```python
from build123d import *

# Parameters (mm, degrees)
F1_DEPTH    = 25
F2_R        = 5
F3_T1_DEPTH = 50.8882578448
F3_T3_DEPTH = 49.1422193702
F4_T1_DEPTH = 50.8882578448
F5_R        = 5


# Not quite as in the source:
# - a fillet or chamfer that OpenCascade refuses, or shapes differently, is made with other operations: its cross-section is extruded or revolved along the edge and cut away or added


with BuildPart() as f1:
    # F0 (on Front) → F1 (new body)
    with BuildSketch(Plane.XZ):
        Polygon((-29.6450223361, 14.0248785508), (-30, 3.8596482585), (-20, 3.8596482585), (-19.6450223361, 14.0248785508), align=None)
        Polygon((-20, 3.8596482585), (-30, 3.8596482585), (-30, -6.1403517415), (17.9300867021, -6.1403517415), (17.9300867021, 3.8596482585), (0, 3.8596482585), (-10, 3.8596482585), align=None)
        Polygon((-9.3028735371, 23.8227382193), (-10, 3.8596482585), (0, 3.8596482585), (0.6971264629, 23.8227382193), align=None)
    extrude(amount=F1_DEPTH)

    # F2
    f2_edges = [f1.edges().sort_by_distance(p)[0] for p in [
        (-29.645022, -12.5, 14.024879),
    ]]
    fillet(f2_edges, radius=F2_R)

    # F3: fillet of radius 5 on 2 edges, made by hand

    # F3_s2 → F3_t1 (cut)
    with BuildSketch(Plane.XZ.offset(-12.9441289224)):
        with BuildLine():
            ThreePointArc((-24.8226739051, 14.0248785508), (-21.2259749034, 12.4981704031), (-19.82571977, 8.8503810672))
            Line((-19.82571977, 8.8503810672), (-19.6450223361, 14.0248785508))
            Line((-19.6450223361, 14.0248785508), (-24.8226739051, 14.0248785508))
        make_face()
    extrude(amount=F3_T1_DEPTH, mode=Mode.SUBTRACT)

    # F3_s4 → F3_t3 (cut)
    with BuildSketch(Plane.XZ.offset(-12.0711096851)):
        with BuildLine():
            ThreePointArc((-9.4713837982, 18.9972357029), (-7.9477215154, 22.419437221), (-4.4744296631, 23.8227382193))
            Line((-4.4744296631, 23.8227382193), (-9.3028735371, 23.8227382193))
            Line((-9.3028735371, 23.8227382193), (-9.4713837982, 18.9972357029))
        make_face()
    extrude(amount=F3_T3_DEPTH, mode=Mode.SUBTRACT)

    # F4: fillet of radius 5 on 1 edges, made by hand

    # F4_s2 → F4_t1 (cut)
    with BuildSketch(Plane.XZ.offset(-12.9441289224)):
        with BuildLine():
            ThreePointArc((-4.4805251061, 23.8227382193), (-0.8838261044, 22.2960300716), (0.516429029, 18.6482407358))
            Line((0.516429029, 18.6482407358), (0.6971264629, 23.8227382193))
            Line((0.6971264629, 23.8227382193), (-4.4805251061, 23.8227382193))
        make_face()
    extrude(amount=F4_T1_DEPTH, mode=Mode.SUBTRACT)

    # F5
    f5_edges = [f1.edges().sort_by_distance(p)[0] for p in [
        (17.930087, -12.5, 3.859648),
    ]]
    fillet(f5_edges, radius=F5_R)


solid = f1.part
```
Verification items for the finished model (mm, model axes). Coordinates: 2 decimals unless noted, no trailing zeros. Loops run counter-clockwise (first coordinate to the right, second up) from the corner with the lowest first, then second, coordinate; pieces in that order, holes last. Notation, with made-up numbers: (-8, 70) - (44, 70) arc R19 ccw to (44, 101) - close; hole circle Ø11 at (-33.75, 23.5). An arc over 180 degrees is marked (long way). Put each result on its own line as item: value.
Item 1: Draft check along X on faces 1 (the face through (-6, -12, -6.14)), 2 (the face through (-15, -12, 3.86)), 3 (the face through (-30, -12, -1)), 4 (the face through (16.43, -12.68, 2.43)). Enter one of: pulls with the +X half, pulls with the -X half, needs draft (parallel to the pull), parting line crosses it, or undercut.
Conclusion:
face 1: needs draft
face 2: undercut
face 3: pulls with the -X half
face 4: pulls with the +X half
Item 2: Section check A-A (y = -9). Enter the section's corners in (x, z).
Conclusion:
outline: (-30, -6.14) - (17.93, -6.14) - (17.93, -1.14) arc R5 ccw to (12.93, 3.86) - (0, 3.86) - (0.52, 18.65) arc R5 ccw to (-4.48, 23.82) arc R5 ccw to (-9.47, 19) - (-10, 3.86) - (-20, 3.86) - (-19.83, 8.85) arc R5 ccw to (-24.82, 14.02) arc R5 ccw to (-29.81, 9.2) - (-30, 3.86) - close
Item 3: Gauge pin test, flat ends, axial feed: pin 1 Ø8 at (x, y) = (-15.5, -10) entering from +Z; pin 2 Ø6 at (x, y) = (-20.5, -19) entering from +Z; pin 3 Ø2 at (x, y) = (-21, -4) entering from +Z. Record the tip position at first contact, or that the pin passes through.
Conclusion:
pin 1: stops at z = 3.86
pin 2: stops at z = 13.85
pin 3: stops at z = 13.15
Item 4: Scan lines: line 1 along X through (y, z) = (-3.75, 4); line 2 along Z through (x, y) = (4.5, -7); line 3 along X through (y, z) = (-21, 7.5). Record each from-to range of solid material in increasing order.
Conclusion:
line 1: x = -30 to -20, -10 to 0
line 2: z = -6.14 to 3.86
line 3: x = -29.87 to -19.87, -9.87 to 0.13
Item 5: Section check C-C (z = 2). Enter the section's corners in (x, y).
Conclusion:
outline: (-30, -25) - (16.82, -25) - (16.82, 0) - (-30, 0) - close
Item 6: Section check B-B (x = -19). Enter the section's corners in (y, z).
Conclusion:
outline: (-25, -6.14) - (0, -6.14) - (0, 3.86) - (-25, 3.86) - close
